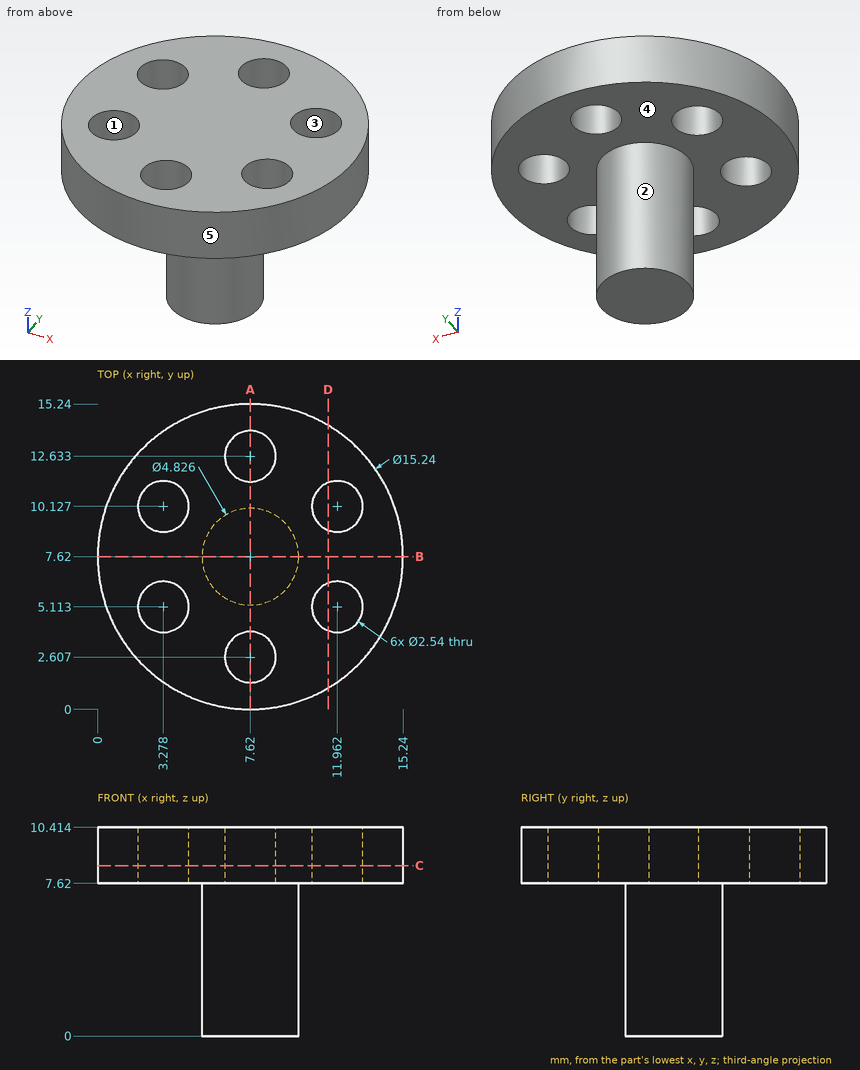
Print and shaded views of the part. All mm, measured from the part's lowest x, y and z. A direction names the side the tool comes from. Give positions to 0.01 mm unless a question says otherwise; leave off trailing zeros. Write each loop counter-clockwise with the first axis right and the second up, starting at its lowest first coordinate (ties: lowest second). Pieces come first, ordered by that corner, then holes. Notation, with made-up numbers: M -26.5,51.25 L 10.5,51.25 A14 cw 10.5,78.25 Z; hole C -24,66.5 d1. An arc over 180 degrees is marked long. Use a Markdown table: item, result.
1) Tool access for the marked faces 1 and 2: list every direction of +Z, -Z, +X, -X, +Y, -Y with a clear straight run to the whole face (end or side of a thin tool).
Responses:
| item | result |
|---|---|
| face 1 | +Z, -Z |
| face 2 | -Z |
2) Cut at A-A (x = 7.62). List the corners of the cut face in (y, z).
Responses:
| item | result |
|---|---|
| outline | M 0,7.62 L 1.34,7.62 L 1.34,10.41 L 0,10.41 Z; M 3.88,7.62 L 5.21,7.62 L 5.21,0 L 10.03,0 L 10.03,7.62 L 11.36,7.62 L 11.36,10.41 L 3.88,10.41 Z; M 13.9,7.62 L 15.24,7.62 L 15.24,10.41 L 13.9,10.41 Z |
3) Cut at B-B (y = 7.62). List the corners of the cut face in (x, z).
Responses:
| item | result |
|---|---|
| outline | M 0,7.62 L 5.21,7.62 L 5.21,0 L 10.03,0 L 10.03,7.62 L 15.24,7.62 L 15.24,10.41 L 0,10.41 Z |
4) Pull direction Y, two halves, no side cores. Call the marked faces 3, 4 and 5: +Y half, -Y half, draft (parallel to the pull), parting line (faces both ways), or undercut.
Responses:
| item | result |
|---|---|
| face 3 | undercut |
| face 4 | draft |
| face 5 | parting line |
5) Cut at C-C (z = 8.5). List the corners of the cut face in (x, y).
Responses:
| item | result |
|---|---|
| outline | C 7.62,7.62 d15.24; hole C 3.28,5.11 d2.54; hole C 3.28,10.13 d2.54; hole C 7.62,2.61 d2.54; hole C 7.62,12.63 d2.54; hole C 11.96,5.11 d2.54; hole C 11.96,10.13 d2.54 |
6) Cut at D-D (x = 11.5). List the corners of the cut face in (y, z).
Responses:
| item | result |
|---|---|
| outline | M 1.06,7.62 L 3.93,7.62 L 3.93,10.41 L 1.06,10.41 Z; M 6.3,7.62 L 8.94,7.62 L 8.94,10.41 L 6.3,10.41 Z; M 11.31,7.62 L 14.18,7.62 L 14.18,10.41 L 11.31,10.41 Z |
7) Drill centre lines: line 1 (Y direction, x = 7.62, z = 9.05); line 2 (Y direction, x = 3, z = 8.5) (1 decimal); line 3 (X direction, y = 4.75, z = 9.25) (1 decimal). Where is each one in solid material? Low to high. Write a range as from..to.
Responses:
| item | result |
|---|---|
| line 1 | y = 0..1.34, 3.88..11.36, 13.9..15.24 |
| line 2 | y = 1.6..3.9, 6.4..8.9, 11.4..13.7 |
| line 3 | x = 0.6..2.1, 4.5..10.7, 13.2..14.7 |
8) Pin check, flat tips, straight feed: pin 1 (6 mm diameter, centred on y = 13.5, z = 3.5, fed in from -X); pin 2 (1.5 mm diameter, centred on y = 3, z = 7, fed in from -X); pin 3 (4 mm diameter, centred on x = 7.62, y = 12.63, fed in from -Z); pin 4 (2 mm diameter, centred on y = 6, z = 6, fed in from +X). Stop position of each tip, or through.
Responses:
| item | result |
|---|---|
| pin 1 | passes through |
| pin 2 | stops at x = 1.26 |
| pin 3 | stops at z = 7.62 |
| pin 4 | stops at x = 9.95 |
